Check sheet for the modelled part. Datum: model origin and axes. Units: mm. A direction names the side the tool comes from. Round coordinates to 2 decimals unless told otherwise and drop trailing zeros. Write each loop counter-clockwise with the first axis right and the second up, starting at its lowest first coordinate (ties: lowest second). Pieces come first, ordered by that corner, then holes. Notation, with made-up numbers: M 47,27.25 L 78,27.25 A12 cw 78,46.25 Z; hole C -1.5,89 d9. An arc over 180 degrees is marked long. One line per item, written item: value.
from build123d import *

# Parameters (mm, degrees)
F0_W     = 368
F0_H     = 722
F1_DEPTH = 19
F2_W     = 368
F2_H     = 19
F3_DEPTH = 5


with BuildPart() as f1:
    # F0 (on Front) → F1 (new body)
    with BuildSketch(Plane.XZ):
        with Locations((184, 361)):
            Rectangle(F0_W, F0_H)
    extrude(amount=F1_DEPTH)

    # F2 (on face) → F3 (cut)
    with BuildSketch(Plane(origin=(0, 0, 0), x_dir=(-1, 0, 0), z_dir=(0, 1, 0))):
        Polygon((-368, 370.5), (-368, 361), (-368, 351.5), (0, 351.5), (0, 361), (0, 370.5), align=None)
        with Locations((-184, 9.5)):
            Rectangle(F2_W, F2_H)
        with Locations((-184, 712.5)):
            Rectangle(F2_W, F2_H)
    extrude(amount=-F3_DEPTH, mode=Mode.SUBTRACT)


solid = f1.part
Q1. Sectioned sample at A-A on x = 296.5. Enter the section's corners in (y, z), and give its area (3 significant figures).
Completed:
outline: M -19,0 L -5,0 L -5,19 L 0,19 L 0,351.5 L -5,351.5 L -5,370.5 L 0,370.5 L 0,703 L -5,703 L -5,722 L -19,722 Z
area: 13,400 mm^2
Q2. Access from +Z, -Z, +X, -X, +Y, -Y to the whole of each face (thin tool, end or side, straight path). Record for faces 4 (the flat face through (368, -9, 356)), 5 (the flat face through (187, -5, 713)), 6 (the flat face through (187, -5, 10)).
Completed:
face 4: +Z, -Z, +X, +Y, -Y
face 5: +Z, +X, -X, +Y
face 6: -Z, +X, -X, +Y
Q3. Scan line: line 1 (Z direction, x = 197.5, y = -3.5). Record every from-to range of solid material in increasing order. Write a range as [from, to].
Completed:
line 1: [19, 351.5], [370.5, 703]
Q4. Draft check along Z on faces 1 (the flat face through (187, -5, 361)), 2 (the flat face through (181, -12, 0)), 3 (the flat face through (0, -9, 356)). Enter one of: pulls with the +Z half, pulls with the -Z half, needs draft (parallel to the pull), parting line crosses it, or undercut.
Completed:
face 1: undercut
face 2: pulls with the -Z half
face 3: needs draft
Q5. Depth check by flat-ended pin: P1, Ø4, axis at x = 192, y = -2.5, coming from the -Z side; P2, Ø1.5, axis at x = 106.5, y = -3.5, coming from the +Z side; P3, Ø5.5, axis at x = 111, z = 5.5, coming from the +Y side. Enter the tip coordinate at first touch or a pass-through.
Completed:
P1: z = 19
P2: z = 703
P3: y = -5
